Verification items for the finished model (mm, model axes). A direction names the side the tool comes from. Give positions to 0.01 mm unless a question says otherwise; leave off trailing zeros. Write each loop counter-clockwise with the first axis right and the second up, starting at its lowest first coordinate (ties: lowest second). Pieces come first, ordered by that corner, then holes. Notation, with made-up numbers: (17.5, -24) - (51.5, -24) arc R28 ccw to (51.5, 13) - close; hole circle Ø11 at (2.5, -27). An arc over 180 degrees is marked (long way). Answer as a JSON object with one key per item and string values. Group by question number.
Item 1: Tool access check on faces 1 (the face through (28.2, 10.68, 0.76)), 2 (the face through (33, 9, 1)), 3 (the face through (1, 13.544, 1)). Record the directions out of +Z, -Z, +X, -X, +Y, -Y that give a thin tool (end or side, any length) a straight path to the whole face; none if there is none.
Item 2: Scan lines: line 1 along Y through (x, z) = (31.5, 0.75); line 2 along X through (y, z) = (9.5, 1.35); line 3 along X through (y, z) = (7.5, 1.4). Record each from-to range of solid material in increasing order. Write a range as [from, to].
Item 3: Draft check along Y on faces 4 (the face through (0, 1, 1)), 5 (the face through (31.83, 7.05, 0.76)), 6 (the face through (1, 9.004, 1)). Enter one of: +Y half, -Y half, draft (parallel to the pull), parting line (faces both ways), or undercut.
Item 4: Sectioned sample at A-A, the plane y = 5.5. Record the boundary of the cut face in (x, z), and give its area (3 significant figures).
```python
from build123d import *

# Parameters (mm, degrees)
SKETCH1_W           = 33
SKETCH1_H           = 17.8
MAIN_BODY_DEPTH     = 1.5
PIN_HOLE_DEPTH      = 1.5
PIN_HOLE_DEPTH_BACK = 10
CUT_EXTRUDE3_DEPTH  = 10


with BuildPart() as part:
    # Sketch1 → Main Body (new body)
    with BuildSketch(Plane.XY):
        with Locations((16.5, 8.9)):
            Rectangle(SKETCH1_W, SKETCH1_H)
    extrude(amount=MAIN_BODY_DEPTH)

    # Sketch7 → Pin Hole (cut, two sides)
    with BuildSketch(Plane(origin=(0, 0, 1.5), x_dir=(-1, 0, 0), z_dir=(0, 0, -1))) as pin_hole_sk:
        with BuildLine():
            Line((0, 16.084169392), (-1.381760133, 16.084169392))
            ThreePointArc((-1.381760133, 16.084169392), (-2.381760133, 15.084169392), (-1.381760133, 14.084169392))
            Line((-1.381760133, 14.084169392), (0, 14.084169392))
            Line((0, 14.084169392), (0, 16.084169392))
        make_face()
        with BuildLine():
            Line((0, 11.544169392), (0, 13.544169392))
            Line((0, 13.544169392), (-1.381760133, 13.544169392))
            ThreePointArc((-1.381760133, 13.544169392), (-2.381760133, 12.544169392), (-1.381760133, 11.544169392))
            Line((-1.381760133, 11.544169392), (0, 11.544169392))
        make_face()
        with BuildLine():
            Line((0, 9.004169392), (0, 11.004169392))
            Line((0, 11.004169392), (-1.381760133, 11.004169392))
            ThreePointArc((-1.381760133, 11.004169392), (-2.381760133, 10.004169392), (-1.381760133, 9.004169392))
            Line((-1.381760133, 9.004169392), (0, 9.004169392))
        make_face()
        with BuildLine():
            Line((0, 6.464169392), (0, 8.464169392))
            Line((0, 8.464169392), (-1.381760133, 8.464169392))
            ThreePointArc((-1.381760133, 8.464169392), (-2.381760133, 7.464169392), (-1.381760133, 6.464169392))
            Line((-1.381760133, 6.464169392), (0, 6.464169392))
        make_face()
        with BuildLine():
            Line((-1.381760133, 3.924169392), (0, 3.924169392))
            Line((0, 3.924169392), (0, 5.924169392))
            Line((0, 5.924169392), (-1.381760133, 5.924169392))
            ThreePointArc((-1.381760133, 5.924169392), (-2.381760133, 4.924169392), (-1.381760133, 3.924169392))
        make_face()
        with BuildLine():
            Line((-1.381760133, 1.384169392), (0, 1.384169392))
            Line((0, 1.384169392), (0, 3.384169392))
            Line((0, 3.384169392), (-1.381760133, 3.384169392))
            ThreePointArc((-1.381760133, 3.384169392), (-2.381760133, 2.384169392), (-1.381760133, 1.384169392))
        make_face()
    extrude(amount=PIN_HOLE_DEPTH, mode=Mode.SUBTRACT)
    extrude(pin_hole_sk.sketch, amount=-PIN_HOLE_DEPTH_BACK, mode=Mode.SUBTRACT)

    # Sketch10 → Cut-Extrude3 (cut)
    with BuildSketch(Plane(origin=(0, 0, 1.5), x_dir=(-1, 0, 0), z_dir=(0, 0, -1))):
        Polygon((-32.45, 7.689172953), (-32.45, 10.078883994), (-31.196454748, 11.3), (-28.806743708, 11.3), (-27.585627701, 10.046454748), (-27.585627701, 7.656743708), (-28.839172953, 6.435627701), (-31.228883994, 6.435627701), align=None)
    extrude(amount=CUT_EXTRUDE3_DEPTH, mode=Mode.SUBTRACT)


solid = part.part
```
Geometry check:
{
 "1": {"face 1": "+Z, -Z", "face 2": "+Z, -Z, +X, +Y, -Y", "face 3": "+Z, -Z, -X"},
 "2": {"line 1": "[0, 6.71], [11, 17.8]", "line 2": "[2.25, 27.59], [32.45, 33]", "line 3": "[2.38, 27.75], [32.27, 33]"},
 "3": {"face 4": "draft", "face 5": "undercut", "face 6": "undercut"},
 "4": {"outline": "(2.2, 0) - (33, 0) - (33, 1.5) - (2.2, 1.5) - close", "area": "46.2 mm^2"}
}
